```python
from build123d import *

# Parameters (mm, degrees)
F0_R     = 32.588749
F1_DEPTH = 88.9
F2_W     = 17.885627
F2_H     = 28.591043
F3_DEPTH = 25.4
F4_R     = 23.990527
F5_DEPTH = 42.545


with BuildPart() as f1:
    # F0 (on Top) → F1 (new body)
    with BuildSketch(Plane.XY):
        Circle(F0_R)
    extrude(amount=F1_DEPTH)

    # F2 (on face) → F3 (join)
    with BuildSketch(Plane.XY.offset(88.9)):
        with Locations((-8.942813, -3.438737)):
            Rectangle(F2_W, F2_H)
    extrude(amount=F3_DEPTH)

    # F4 (on Right) → F5 (cut, symmetric)
    with BuildSketch(Plane.YZ):
        with Locations((0, 42.958003)):
            Circle(F4_R)
    extrude(amount=F5_DEPTH, both=True, mode=Mode.SUBTRACT)


solid = f1.part
```
Could you check a few things on this model? Use its own coordinates, in mm. A direction names the side the tool comes from. Round coordinates to 2 decimals unless told otherwise and drop trailing zeros. Loops run counter-clockwise (first coordinate to the right, second up) from the corner with the lowest first, then second, coordinate; pieces in that order, holes last. Notation, with made-up numbers: (6.5, 62.25) - (23.5, 62.25) arc R24 ccw to (23.5, 95.25) - close; hole circle Ø3 at (33, 76). An arc over 180 degrees is marked (long way). Answer in a Markdown table with one row per item. Add a question column.
(1) I need wall thicknesses on line 1 along Z through (x, y) = (-14, 0); line 2 along Y through (x, z) = (-11, 94); line 3 along Z through (x, y) = (7, -15). Which ranges of each line are inside material? Lowest first, please.
(2) If we mould it in two halves opening along Y, with no side actions, what happens to faces 5 (the face through (17.52, 27.48, 43.83)), 6 (the face through (0.456, 22.883, 50.164)), 7 (the face through (-9, 10.857, 101))? For each: pulls with the +Y half, pulls with the -Y half, needs draft (parallel to the pull), parting line crosses it, or undercut.
(3) If we section it at B-B (x = -14.5): Please give me the cut outline in (y, z), plus the area to 3 significant figures.
(4) For faces 1 (the face through (-17.886, -4, 101)), 2 (the face through (0, 0, 0)), 3 (the face through (0, -4, 101)), 4 (the face through (-9, -17.734, 101)), which set-ups out of +Z, -Z, +X, -X, +Y, -Y let a thin tool reach every point of the face, with its end or its side?
(5) If we section it at C-C (y = -7): Please give me the cut outline in (x, z).
(6) If we section it at D-D (x = 19): Please give me the cut outline in (y, z).
(7) If we section it at A-A (y = 0): Please give me the cut outline in (x, z).
(8) I'm going to push flat-ended pins straight in: pin 1 (4 mm diameter, centred on y = -22, z = 13, fed in from +X); pin 2 (1 mm diameter, centred on x = 20, z = 65.5, fed in from +Y); pin 3 (1.5 mm diameter, centred on x = -2.5, z = 94.5, fed in from -Y); pin 4 (1 mm diameter, centred on x = -17, y = -1, fed in from -Z). Where does each tip first touch, or does it pass through?
Model answer:
| question | item | result |
|---|---|---|
| 1 | line 1 | z = 0 to 18.97, 66.95 to 114.3 |
| 1 | line 2 | y = -17.73 to 10.86 |
| 1 | line 3 | z = 0 to 24.24, 61.68 to 88.9 |
| 2 | face 5 | parting line crosses it |
| 2 | face 6 | undercut |
| 2 | face 7 | pulls with the +Y half |
| 3 | outline | (-29.19, 0) - (29.19, 0) - (29.19, 88.9) - (10.86, 88.9) - (10.86, 114.3) - (-17.73, 114.3) - (-17.73, 88.9) - (-29.19, 88.9) - close; hole circle Ø47.98 at (0, 42.96) |
| 3 | area | 4,110 mm² |
| 4 | face 1 | +Z, -X, +Y, -Y |
| 4 | face 2 | -Z, +X, -X, +Y, -Y |
| 4 | face 3 | +Z, +X, +Y, -Y |
| 4 | face 4 | +Z, +X, -X, -Y |
| 5 | outline | (-31.83, 0) - (31.83, 0) - (31.83, 20.01) - (-31.83, 20.01) - close; (-31.83, 65.9) - (31.83, 65.9) - (31.83, 88.9) - (0, 88.9) - (0, 114.3) - (-17.89, 114.3) - (-17.89, 88.9) - (-31.83, 88.9) - close |
| 6 | outline | (-26.48, 0) - (26.48, 0) - (26.48, 88.9) - (-26.48, 88.9) - close; hole circle Ø47.98 at (0, 42.96) |
| 7 | outline | (-32.59, 0) - (32.59, 0) - (32.59, 18.97) - (-32.59, 18.97) - close; (-32.59, 66.95) - (32.59, 66.95) - (32.59, 88.9) - (0, 88.9) - (0, 114.3) - (-17.89, 114.3) - (-17.89, 88.9) - (-32.59, 88.9) - close |
| 8 | pin 1 | stops at x = 25.73 |
| 8 | pin 2 | stops at y = 26.11 |
| 8 | pin 3 | stops at y = -17.73 |
| 8 | pin 4 | stops at z = 0 |
